Work out the finished part from the listing and answer in its coordinate system (mm). A direction names the side the tool comes from. Give positions to 0.01 mm unless a question says otherwise; leave off trailing zeros. Loops run counter-clockwise (first coordinate to the right, second up) from the corner with the lowest first, then second, coordinate; pieces in that order, holes last. Notation, with made-up numbers: (32.5, 4.25) - (86.5, 4.25) arc R19 ccw to (86.5, 26.25) - close; hole circle Ø6 at (11.5, 48). An arc over 180 degrees is marked (long way). One line per question, with ' | ' between items. Start each with the question number.
1. Find the intervals of material crossed by line 1 (Z direction, x = -127, y = 0.9); line 2 (X direction, y = 0.3, z = 68); line 3 (Z direction, x = 87.5, y = 1.4), in increasing order.
2. Which of the six approach directions +Z, -Z, +X, -X, +Y, -Y give full straight-line access (tool end or side, diameter ignored) to faces 5 (the face through (30, 3, 3)), 6 (the face through (13.22, 1.52, -29.48))?
3. Section C-C (x = -78) is taken. Determine the outline of the cut face in (y, z).
4. Section D-D (z = 8) is taken. Determine the outline of the cut face in (x, y).
5. Section B-B (z = 88) is taken. Determine the outline of the cut face in (x, y).
6. Section A-A (x = 194) is taken. Determine the outline of the cut face in (y, z).
7. For a pull along X with two mould halves and no side action, classify faces 1 (the face through (225.365, 1.479, -134.918)), 2 (the face through (43.32, 1.48, -164.21)), 3 (the face through (-29.666, 1.521, 19.82)), 4 (the face through (108.04, 1.48, -112.7)) as released by +X, released by -X, zero draft, split by the parting line, or undercut.
8. Each of these flat-tipped pins is pushed along its axis until it touches: pin 1 (0.9 mm diameter, centred on y = 2, z = 65, fed in from +X); pin 2 (10 mm diameter, centred on x = 99.57, z = 185.65, fed in from +Y); pin 3 (1.5 mm diameter, centred on x = 87, y = 1, fed in from -Z); pin 4 (1.5 mm diameter, centred on x = 75, y = 2, fed in from +Z). Where does it stop, or does it pass through?
from build123d import *

# Parameters (mm, degrees)
SKETCH1_R             = 1.75
BOSS_EXTRUDE2_DEPTH   = 3
SKETCH1_R_2           = 4.25
SKETCH1_R_3           = 10.5
BOSS_EXTRUDE2_2_DEPTH = 3
MIRROR1_OUTLINE_R     = 1.75
MIRROR1_OUTLINE_R_2   = 4.25
MIRROR1_OUTLINE_R_3   = 10.5
MIRROR1_DEPTH         = 3
FILLET1_R             = 10
SKETCH2_R             = 17.5
CUT_EXTRUDE1_DEPTH    = 10


# Read off the part's stored shape, not the designer's step: Mirror1
with BuildPart() as part:
    # Sketch1 → Boss-Extrude2 (new body)
    with BuildSketch(Plane(origin=(0, 0, 0), x_dir=(1, 0, 0), z_dir=(0, 1, 0))):
        with Locations(Location((153.848996294, -160.649182064, 0), (0, 0, 270))):
            Circle(SKETCH1_R)
    extrude(amount=BOSS_EXTRUDE2_DEPTH)



with BuildPart() as body_2:
    # Sketch1 → Boss-Extrude2 2 (new body)
    with BuildSketch(Plane(origin=(0, 0, 0), x_dir=(1, 0, 0), z_dir=(0, 1, 0))):
        with BuildLine():
            Line((-160.429103157, 154.350817936), (-0.429103157, 154.350817936))
            Line((-0.429103157, 154.350817936), (88.320896843, 174.350817936))
            ThreePointArc((88.320896843, 174.350817936), (99.570896843, 185.600817936), (110.820896843, 174.350817936))
            Line((110.820896843, 174.350817936), (199.570896843, 160.150817936))
            ThreePointArc((199.570896843, 160.150817936), (225.370896843, 134.350817936), (199.570896843, 108.550817936))
            Line((199.570896843, 108.550817936), (199.570896843, -5.649182064))
            Line((199.570896843, -5.649182064), (140.384809243, -5.649182064))
            Line((140.384809243, -5.649182064), (17.871310963, -5.649182064))
            Line((17.871310963, -5.649182064), (-17.871310963, -5.649182064))
            Line((-17.871310963, -5.649182064), (-140.384809243, -5.649182064))
            Line((-140.384809243, -5.649182064), (-160.429103157, -5.649182064))
            Line((-160.429103157, -5.649182064), (-160.429103157, 154.350817936))
        make_face()
        with Locations(Location((99.570896843, 174.350817936, 0), (0, 0, 270))):
            Circle(SKETCH1_R_2, mode=Mode.SUBTRACT)
        with Locations(Location((199.570896843, 134.350817936, 0), (0, 0, 270))):
            Circle(SKETCH1_R_3, mode=Mode.SUBTRACT)
        with Locations(Location((-155.429103157, 149.350817936, 0), (0, 0, 270))):
            Circle(SKETCH1_R, mode=Mode.SUBTRACT)
        with Locations(Location((153.848996294, 149.350817936, 0), (0, 0, 270))):
            Circle(SKETCH1_R, mode=Mode.SUBTRACT)
        with Locations(Location((107.320896843, 174.350817936, 0), (0, 0, 270))):
            Circle(SKETCH1_R, mode=Mode.SUBTRACT)
        with Locations(Location((91.820896843, 174.350817936, 0), (0, 0, 270))):
            Circle(SKETCH1_R, mode=Mode.SUBTRACT)
        with Locations(Location((99.570896843, 182.100817936, 0), (0, 0, 270))):
            Circle(SKETCH1_R, mode=Mode.SUBTRACT)
        with BuildLine():
            Line((98.615479423, 119.350817936), (7.5, 119.350817936))
            Line((7.5, 119.350817936), (7.5, 16.506675056))
            Line((7.5, 16.506675056), (105.19311723, 101.818575184))
            ThreePointArc((105.19311723, 101.818575184), (107.978236162, 112.863478785), (98.615479423, 119.350817936))
        make_face(mode=Mode.SUBTRACT)
        with BuildLine():
            Line((-102.646063409, 98.639396028), (-7.5, 16.39642362))
            Line((-7.5, 16.39642362), (-7.5, 119.350817936))
            Line((-7.5, 119.350817936), (-94.935387285, 119.350817936))
            ThreePointArc((-94.935387285, 119.350817936), (-105.985472395, 111.673646608), (-102.646063409, 98.639396028))
        make_face(mode=Mode.SUBTRACT)
        with BuildLine():
            Line((122.271358487, 96.81800419), (13.521694655, 1.850817936))
            Line((13.521694655, 1.850817936), (138.848996294, 1.850817936))
            Line((138.848996294, 1.850817936), (138.848996294, 89.285761438))
            ThreePointArc((138.848996294, 89.285761438), (132.985638769, 98.390056525), (122.271358487, 96.81800419))
        make_face(mode=Mode.SUBTRACT)
        with BuildLine():
            Line((-119.347301526, 94.437659895), (-12.234519996, 1.850817936))
            Line((-12.234519996, 1.850817936), (-138.848996294, 1.850817936))
            Line((-138.848996294, 1.850817936), (-138.848996294, 85.517256632))
            ThreePointArc((-138.848996294, 85.517256632), (-131.96263843, 96.23977608), (-119.347301526, 94.437659895))
        make_face(mode=Mode.SUBTRACT)
    extrude(amount=BOSS_EXTRUDE2_2_DEPTH)


with BuildPart() as part_1:
    add(part.part)

    add(body_2.part)  # Mirror1 merges body 2
    # Mirror1 outline → Mirror1 (add)
    # profile 1 of 2: a face of its own
    with BuildSketch(Plane(origin=(0, 0, 0), x_dir=(1, 0, 0), z_dir=(0, 1, 0))):
        with BuildLine():
            Line((-160.429103157, -5.649182064), (-160.429103157, -165.649182064))
            Line((-160.429103157, -165.649182064), (-0.429103157, -165.649182064))
            Line((-0.429103157, -165.649182064), (88.320896843, -185.649182064))
            ThreePointArc((88.320896843, -185.649182064), (99.570896843, -196.899182064), (110.820896843, -185.649182064))
            Line((110.820896843, -185.649182064), (199.570896843, -171.449182064))
            ThreePointArc((199.570896843, -171.449182064), (225.370896843, -145.649182064), (199.570896843, -119.849182064))
            Line((199.570896843, -119.849182064), (199.570896843, -5.649182064))
            Line((199.570896843, -5.649182064), (-160.429103157, -5.649182064))
        make_face()
        with Locations((-155.429103157, -160.649182064)):
            Circle(MIRROR1_OUTLINE_R, mode=Mode.SUBTRACT)
        with BuildLine():
            Line((-138.848996294, -96.81562076), (-138.848996294, -13.149182064))
            Line((-138.848996294, -13.149182064), (-12.234519996, -13.149182064))
            Line((-12.234519996, -13.149182064), (-119.347301526, -105.736024024))
            ThreePointArc((-119.347301526, -105.736024024), (-131.96263843, -107.538140208), (-138.848996294, -96.81562076))
        make_face(mode=Mode.SUBTRACT)
        with BuildLine():
            Line((-7.5, -27.694787748), (-7.5, -130.649182064))
            Line((-7.5, -130.649182064), (-94.935387285, -130.649182064))
            ThreePointArc((-94.935387285, -130.649182064), (-105.985472395, -122.972010736), (-102.646063409, -109.937760156))
            Line((-102.646063409, -109.937760156), (-7.5, -27.694787748))
        make_face(mode=Mode.SUBTRACT)
        with Locations((99.570896843, -193.399182064)):
            Circle(MIRROR1_OUTLINE_R, mode=Mode.SUBTRACT)
        with Locations((91.820896843, -185.649182064)):
            Circle(MIRROR1_OUTLINE_R, mode=Mode.SUBTRACT)
        with Locations((99.570896843, -185.649182064)):
            Circle(MIRROR1_OUTLINE_R_2, mode=Mode.SUBTRACT)
        with Locations((107.320896843, -185.649182064)):
            Circle(MIRROR1_OUTLINE_R, mode=Mode.SUBTRACT)
        with Locations((153.848996294, -160.649182064)):
            Circle(MIRROR1_OUTLINE_R, mode=Mode.SUBTRACT)
        with Locations((199.570896843, -145.649182064)):
            Circle(MIRROR1_OUTLINE_R_3, mode=Mode.SUBTRACT)
        with BuildLine():
            Line((98.615479423, -130.649182064), (7.5, -130.649182064))
            Line((7.5, -130.649182064), (7.5, -27.805039185))
            Line((7.5, -27.805039185), (105.19311723, -113.116939312))
            ThreePointArc((105.19311723, -113.116939312), (107.978236162, -124.161842913), (98.615479423, -130.649182064))
        make_face(mode=Mode.SUBTRACT)
        with BuildLine():
            Line((138.848996294, -13.149182064), (138.848996294, -100.584125566))
            ThreePointArc((138.848996294, -100.584125566), (132.985638769, -109.688420653), (122.271358487, -108.116368318))
            Line((122.271358487, -108.116368318), (13.521694655, -13.149182064))
            Line((13.521694655, -13.149182064), (138.848996294, -13.149182064))
        make_face(mode=Mode.SUBTRACT)
    # profile 2 of 2: a face of its own
    with BuildSketch(Plane(origin=(0, 0, 0), x_dir=(1, 0, 0), z_dir=(0, 1, 0))):
        with Locations((153.848996294, 149.350817936)):
            Circle(MIRROR1_OUTLINE_R)
    extrude(amount=MIRROR1_DEPTH)

    # Fillet1
    fillet1_edges = [part_1.edges().sort_by_distance(p)[0] for p in [
        (7.5, 1.5, 27.805039185),
        (13.521694655, 1.5, 13.149182064),
        (-7.5, 1.5, 27.694787748),
        (-12.234519996, 1.5, 13.149182064),
        (7.5, 1.5, -16.506675056),
        (13.521694655, 1.5, -1.850817936),
        (-7.5, 1.5, -16.39642362),
        (-12.234519996, 1.5, -1.850817936),
    ]]
    fillet(fillet1_edges, radius=FILLET1_R)

    # Sketch2 → Cut-Extrude1 (cut)
    with BuildSketch(Plane(origin=(0, 3, 0), x_dir=(1, 0, 0), z_dir=(0, 1, 0))):
        with Locations(Location((0, -5.649182064, 0), (0, 0, 270))):
            Circle(SKETCH2_R)
    extrude(amount=-CUT_EXTRUDE1_DEPTH, mode=Mode.SUBTRACT)


solid = part_1.part
Conclusion:
1) line 1: -154.35 to -97.31, -1.85 to 13.15, 108.61 to 165.65 | line 2: -160.43 to -138.85, -75.69 to -54.13, -7.5 to 7.5, 53.53 to 76.33, 138.85 to 199.57 | line 3: -174.17 to -119.35, -86.37 to -66.45, -1.85 to 13.15, 77.75 to 97.67, 130.65 to 185.46
2) face 5: +Z, -Z, +X, -X, +Y | face 6: +Y, -Y
3) outline: (0, -154.35) - (3, -154.35) - (3, -119.35) - (0, -119.35) - close; (0, -77.34) - (3, -77.34) - (3, -58.7) - (0, -58.7) - close; (0, -1.85) - (3, -1.85) - (3, 13.15) - (0, 13.15) - close; (0, 70) - (3, 70) - (3, 88.63) - (0, 88.63) - close; (0, 130.65) - (3, 130.65) - (3, 165.65) - (0, 165.65) - close
4) outline: (-160.43, 0) - (-17.34, 0) - (-17.34, 3) - (-160.43, 3) - close; (17.34, 0) - (199.57, 0) - (199.57, 3) - (17.34, 3) - close
5) outline: (-160.43, 0) - (-138.85, 0) - (-138.85, 3) - (-160.43, 3) - close; (-98.83, 0) - (-77.27, 0) - (-77.27, 3) - (-98.83, 3) - close; (-7.5, 0) - (7.5, 0) - (7.5, 3) - (-7.5, 3) - close; (76.43, 0) - (99.24, 0) - (99.24, 3) - (76.43, 3) - close; (138.85, 0) - (199.57, 0) - (199.57, 3) - (138.85, 3) - close
6) outline: (0, -161.04) - (3, -161.04) - (3, -143.25) - (0, -143.25) - close; (0, -125.45) - (3, -125.45) - (3, 136.75) - (0, 136.75) - close; (0, 154.55) - (3, 154.55) - (3, 172.34) - (0, 172.34) - close
7) face 1: released by +X | face 2: released by -X | face 3: undercut | face 4: undercut
8) pin 1: x = 199.57 | pin 2: y = 3 | pin 3: z = -174.22 | pin 4: z = 182.82
